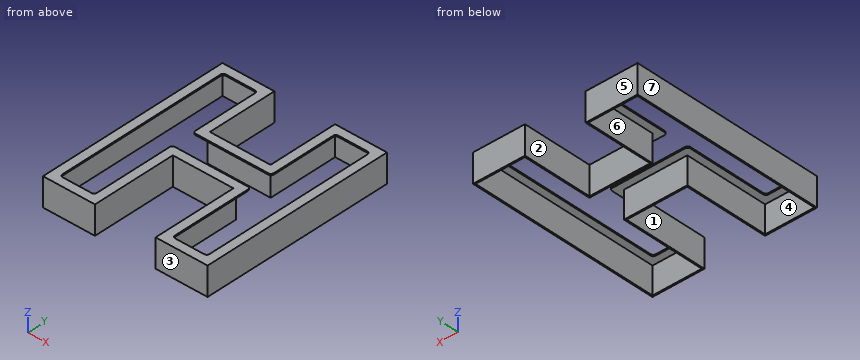
from build123d import *

# Parameters (mm, degrees)
BOSS_EXTRUDE1_DEPTH      = 1
BOSS_EXTRUDE1_DEPTH_BACK = 20
CUT_EXTRUDE1_DEPTH       = 3814.653559302
CUT_EXTRUDE2_DEPTH       = 20
FILLET1_R                = 2


with BuildPart() as part:
    # Sketch1 → Boss-Extrude1 (new, two sides: drawn at the far end of the back side and taken through both)
    with BuildSketch(Plane.XY.offset(-BOSS_EXTRUDE1_DEPTH_BACK)):
        Polygon((3401.843352704, -1645.582577839), (3440.286390679, -1645.582577839), (3440.286390679, -1502.582577839), (3401.843352704, -1502.582577839), (3401.843352704, -1553.974982902), (3356.995251438, -1553.974982902), (3356.995251438, -1502.582577839), (3318.552213464, -1502.582577839), (3318.552213464, -1645.582577839), (3356.995251438, -1645.582577839), (3356.995251438, -1583.557261383), (3401.843352704, -1583.557261383), align=None)
    extrude(amount=BOSS_EXTRUDE1_DEPTH + BOSS_EXTRUDE1_DEPTH_BACK)

    # Sketch2 → Cut-Extrude1 (cut, through all)
    with BuildSketch(Plane.XY.offset(1)):
        Polygon((3408.343352704, -1577.057261383), (3408.343352704, -1639.082577839), (3433.786390679, -1639.082577839), (3433.786390679, -1509.082577839), (3408.343352704, -1509.082577839), (3408.343352704, -1560.474982902), (3350.495251438, -1560.474982902), (3350.495251438, -1509.082577839), (3325.052213464, -1509.082577839), (3325.052213464, -1639.082577839), (3350.495251438, -1639.082577839), (3350.495251438, -1577.057261383), align=None)
    extrude(amount=-CUT_EXTRUDE1_DEPTH, mode=Mode.SUBTRACT)

    # Sketch3 → Cut-Extrude2 (cut)
    with BuildSketch(Plane(origin=(0, 0, -20), x_dir=(-1, 0, 0), z_dir=(0, 0, -1))):
        Polygon((-3402.843352704, -1644.582577839), (-3402.843352704, -1582.557261383), (-3355.995251438, -1582.557261383), (-3355.995251438, -1644.582577839), (-3319.552213464, -1644.582577839), (-3319.552213464, -1503.582577839), (-3355.995251438, -1503.582577839), (-3355.995251438, -1554.974982902), (-3402.843352704, -1554.974982902), (-3402.843352704, -1503.582577839), (-3439.286390679, -1503.582577839), (-3439.286390679, -1644.582577839), align=None)
    extrude(amount=-CUT_EXTRUDE2_DEPTH, mode=Mode.SUBTRACT)

    # Fillet1
    fillet1_edges = [part.edges().sort_by_distance(p)[0] for p in [
        (3408.343352704, -1639.082577839, 0.5),
        (3408.343352704, -1577.057261383, 0.5),
        (3433.786390679, -1639.082577839, 0.5),
        (3433.786390679, -1509.082577839, 0.5),
        (3408.343352704, -1509.082577839, 0.5),
        (3408.343352704, -1560.474982902, 0.5),
        (3350.495251438, -1560.474982902, 0.5),
        (3350.495251438, -1509.082577839, 0.5),
        (3325.052213464, -1509.082577839, 0.5),
        (3325.052213464, -1639.082577839, 0.5),
        (3350.495251438, -1639.082577839, 0.5),
        (3350.495251438, -1577.057261383, 0.5),
    ]]
    fillet(fillet1_edges, radius=FILLET1_R)


solid = part.part
Geometry: final body of the model. Coordinates: model frame, mm. Face numbers are marked on the shaded views. A direction names the side the tool comes from. Give positions to 0.01 mm unless a question says otherwise; leave off trailing zeros. Order: outer loops, then holes, each group sorted by start corner. A loop starts at its lowest first (then second) coordinate and runs counter-clockwise, first axis right, second up. Notation, with made-up numbers: (32, -1) - (63, -1) arc R18 cw to (63, 29) - close; hole circle Ø9 at (5.25, -21.75). An arc over 180 degrees is marked (long way). Use CSV: the item, a comma, the result in double quotes.
1. Section query B-B (z = -3.25). Output: boundary loops of the cut face in (x, y), plus the area to 3 significant figures.
Answers below:
outline,"(3318.55, -1645.58) - (3357, -1645.58) - (3357, -1583.56) - (3401.84, -1583.56) - (3401.84, -1645.58) - (3440.29, -1645.58) - (3440.29, -1502.58) - (3401.84, -1502.58) - (3401.84, -1553.97) - (3357, -1553.97) - (3357, -1502.58) - (3318.55, -1502.58) - close; hole (3319.55, -1644.58) - (3356, -1644.58) - (3356, -1582.56) - (3402.84, -1582.56) - (3402.84, -1644.58) - (3439.29, -1644.58) - (3439.29, -1503.58) - (3402.84, -1503.58) - (3402.84, -1554.97) - (3356, -1554.97) - (3356, -1503.58) - (3319.55, -1503.58) - close"
area,"752 mm2"
2. Access query for the marked faces 1, 2, 3 and 4. Directions: +Z, -Z, +X, -X, +Y, -Y. A direction counts if a zero-diameter tool reaches every point of the face in a straight line with its end or side. Return the directions, or none.
Answers below:
face 1,"+Z, -Z, -Y"
face 2,"+Z, -Z, +Y"
face 3,"+Z, -Z, +X, -X, -Y"
face 4,"-Z"
3. Section query C-C (y = -1574.5). Output: boundary loops of the cut face in (x, z).
Answers below:
outline,"(3318.55, -20) - (3319.55, -20) - (3319.55, 0) - (3325.05, 0) - (3325.05, 1) - (3318.55, 1) - close; (3433.79, 0) - (3439.29, 0) - (3439.29, -20) - (3440.29, -20) - (3440.29, 1) - (3433.79, 1) - close"
4. Material intervals for line 1 along X through (y, z) = (-1605.5, -6); line 2 along Y through (x, z) = (3327.5, -10.75); line 3 along X through (y, z) = (-1583, -17.75), sorted ascending. Write a range as from..to.
Answers below:
line 1,"3318.55..3319.55, 3356..3357, 3401.84..3402.84, 3439.29..3440.29"
line 2,"-1645.58..-1644.58, -1503.58..-1502.58"
line 3,"3318.55..3319.55, 3356..3402.84, 3439.29..3440.29"
5. Mould query, pull axis X, two halves, no side actions, for the marked faces 5, 6 and 7. Classes: +X half, -X half, draft (parallel to the pull), parting line (faces both ways), or undercut.
Answers below:
face 5,"draft"
face 6,"undercut"
face 7,"-X half"
6. Contact query for flat-ended pins moving along their axis: pin 1 (1 mm diameter, centred on x = 3353.5, y = -1621.5, fed in from -Z); pin 2 (1.1 mm diameter, centred on x = 3374.5, z = 0.5, fed in from +Y) (3 decimals); pin 3 (10 mm diameter, centred on x = 3331, y = -1601, fed in from +Z). Output: stop coordinate, or through.
Answers below:
pin 1,"z = 0"
pin 2,"y = -1553.975"
pin 3,"through"
7. Section query D-D (x = 3397). Output: boundary loops of the cut face in (y, z).
Answers below:
outline,"(-1583.56, -20) - (-1582.56, -20) - (-1582.56, 0) - (-1577.06, 0) - (-1577.06, 1) - (-1583.56, 1) - close; (-1560.47, 0) - (-1554.97, 0) - (-1554.97, -20) - (-1553.97, -20) - (-1553.97, 1) - (-1560.47, 1) - close"
8. Section query A-A (y = -1621). Output: boundary loops of the cut face in (x, z).
Answers below:
outline,"(3318.55, -20) - (3319.55, -20) - (3319.55, 0) - (3325.05, 0) - (3325.05, 1) - (3318.55, 1) - close; (3350.5, 0) - (3356, 0) - (3356, -20) - (3357, -20) - (3357, 1) - (3350.5, 1) - close; (3401.84, -20) - (3402.84, -20) - (3402.84, 0) - (3408.34, 0) - (3408.34, 1) - (3401.84, 1) - close; (3433.79, 0) - (3439.29, 0) - (3439.29, -20) - (3440.29, -20) - (3440.29, 1) - (3433.79, 1) - close"
